The listing builds one solid part. Answer for the finished solid, in the listing's coordinates (mm). Round coordinates to 2 decimals unless told otherwise and drop trailing zeros. Order: outer loops, then holes, each group sorted by start corner. A loop starts at its lowest first (then second) coordinate and runs counter-clockwise, first axis right, second up. Notation, with made-up numbers: M 75,-3.5 L 130,-3.5 A23 ccw 130,4.5 Z; hole C 26,-25 d5. An arc over 180 degrees is marked long. Write item = value, one per line. Start each with the question number.
(1) A cutting plane is placed at C-C, the plane z = -1. Determine the outline of the cut face in (x, y), and give its area (3 significant figures).
(2) A cutting plane is placed at A-A, the plane x = 0. Determine the outline of the cut face in (y, z) (3 decimals), and give its area (3 significant figures).
(3) A cutting plane is placed at D-D, the plane z = 2. Determine the outline of the cut face in (x, y), and give its area (3 significant figures).
(4) Each of these flat-tipped pins is pushed along its axis until it touches: pin 1 (6 mm diameter, centred on x = 0, y = 0, fed in from +Z); pin 2 (3 mm diameter, centred on x = -5, z = -2, fed in from -Y). Where does it stop, or does it pass through?
(5) For a pull along X with two mould halves and no side action, classify faces 1 (the face through (2, 5, 0)), 2 (the face through (3.05, -1.26, 0.23)), 3 (the face through (-1.08, -4.88, 1.57)) as released by +X, released by -X, zero draft, split by the parting line, or undercut.
(6) Straight lines are drawn through the part: probe 1 along Y at (x, z) = (0, 1.55); probe 2 along Z at (x, y) = (-4, 5) (3 decimals); probe 3 along X at (y, z) = (3, -1.25). For each, find the intervals that lie inside material, in ascending order. Write a range as from..to.
from build123d import *

# Parameters (mm, degrees)
F0_R     = 5
F1_DEPTH = 3.175
F2_R     = 7.62
F2_R_2   = 5
F3_DEPTH = 3.175
F4_R     = 3.302
F5_DEPTH = 6.351
F6_SIZE  = 0.381


with BuildPart() as f1:
    # F0 (on Top) → F1 (new body)
    with BuildSketch(Plane.XY):
        Circle(F0_R)
    extrude(amount=F1_DEPTH)

    # F2 (on face) → F3 (join)
    with BuildSketch(Plane(origin=(0, 0, 0), x_dir=(1, 0, 0), z_dir=(0, 0, -1))):
        Circle(F2_R)
        Circle(F2_R_2, mode=Mode.SUBTRACT)
        Circle(F2_R_2)
    extrude(amount=F3_DEPTH)

    # F4 (on face) → F5 (cut, through all)
    with BuildSketch(Plane.XY.offset(3.175)):
        Circle(F4_R)
    extrude(amount=-F5_DEPTH, mode=Mode.SUBTRACT)

    # F6
    f6_edges = [f1.edges().sort_by_distance(p)[0] for p in [
        (-3.302, 0, -3.175),
    ]]
    chamfer(f6_edges, length=F6_SIZE)


solid = f1.part
Reported:
q1.outline = C 0,0 d15.24; hole C 0,0 d6.6
q1.area = 148 mm²
q2.outline = M -7.62,-3.175 L -3.683,-3.175 L -3.302,-2.794 L -3.302,3.175 L -5,3.175 L -5,0 L -7.62,0 Z; M 3.302,-2.794 L 3.683,-3.175 L 7.62,-3.175 L 7.62,0 L 5,0 L 5,3.175 L 3.302,3.175 Z
q2.area = 38.1 mm²
q3.outline = C 0,0 d10; hole C 0,0 d6.6
q3.area = 44.3 mm²
q4.pin_1 = through
q4.pin_2 = -6.77
q5.face_1 = zero draft
q5.face_2 = undercut
q5.face_3 = split by the parting line
q6.probe_1 = -5..-3.3, 3.3..5
q6.probe_2 = -3.175..0
q6.probe_3 = -7..-1.38, 1.38..7
